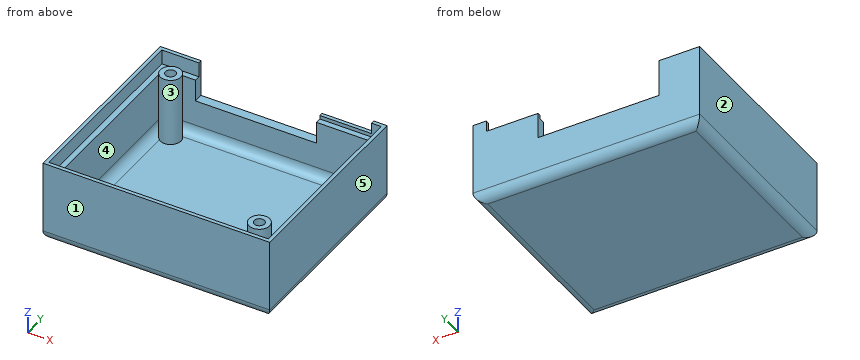
from build123d import *

# Parameters (mm, degrees)
F0_W        = 56.3
F0_H        = 48.55
F0_R        = 2.8
F1_DEPTH    = 2.5
F0_W_2      = 59.4
F0_H_2      = 51.65
F2_DEPTH    = 18
F0_W_3      = 61.4
F0_H_3      = 53.65
F3_DEPTH    = 22
F0_R_2      = 1.4
F4_DEPTH    = 21
F5_DEPTH    = 15
F6_T1_DEPTH = 48.55
F6_T3_DEPTH = 56.3
F6_T5_DEPTH = 73.9
F6_T7_DEPTH = 66.15
F7_W        = 32.75
F7_H        = 1
F7_H_2      = 1.55
F8_DEPTH    = 10
F7_W_2      = 14
F9_DEPTH    = 3


# Not quite as in the source:
# - a fillet or chamfer that OpenCascade refuses, or shapes differently, is made with other operations: its cross-section is extruded or revolved along the edge and cut away or added


with BuildPart() as f1:
    # F0 (on Top) → F1 (new body)
    with BuildSketch(Plane.XY):
        Rectangle(F0_W, F0_H)
        with Locations((23.88, -20.035)):
            Circle(F0_R, mode=Mode.SUBTRACT)
        with Locations((-23.91, 20.085)):
            Circle(F0_R, mode=Mode.SUBTRACT)
    extrude(amount=F1_DEPTH)

    # F0 (on Top) → F2 (join)
    with BuildSketch(Plane.XY):
        Rectangle(F0_W_2, F0_H_2)
        Rectangle(F0_W, F0_H, mode=Mode.SUBTRACT)
    extrude(amount=F2_DEPTH)

    # F0 (on Top) → F3 (join)
    with BuildSketch(Plane.XY):
        Rectangle(F0_W_3, F0_H_3)
        Rectangle(F0_W_2, F0_H_2, mode=Mode.SUBTRACT)
    extrude(amount=F3_DEPTH)

    # F0 (on Top) → F4 (join)
    with BuildSketch(Plane.XY):
        with Locations((-23.91, 20.085)):
            Circle(F0_R)
        with Locations((-23.91, 20.085)):
            Circle(F0_R_2, mode=Mode.SUBTRACT)
        with Locations((23.88, -20.035)):
            Circle(F0_R)
        with Locations((23.88, -20.035)):
            Circle(F0_R_2, mode=Mode.SUBTRACT)
    extrude(amount=F4_DEPTH)

    # F0 (on Top) → F5 (join)
    with BuildSketch(Plane.XY):
        with Locations((23.88, -20.035)):
            Circle(F0_R_2)
        with Locations((-23.91, 20.085)):
            Circle(F0_R_2)
    extrude(amount=F5_DEPTH)

    # F6: fillet of radius 2.5 on 8 edges, made by hand

    # F6_s2 → F6_t1 (join)
    with BuildSketch(Plane.XZ.offset(-24.275)):
        with BuildLine():
            ThreePointArc((28.15, 5), (27.417766953, 3.232233047), (25.65, 2.5))
            Line((25.65, 2.5), (28.15, 2.5))
            Line((28.15, 2.5), (28.15, 5))
        make_face()
        with BuildLine():
            ThreePointArc((-28.15, 5), (-27.417766953, 3.232233047), (-25.65, 2.5))
            Line((-25.65, 2.5), (-28.15, 2.5))
            Line((-28.15, 2.5), (-28.15, 5))
        make_face()
    extrude(amount=F6_T1_DEPTH)

    # F6_s4 → F6_t3 (join)
    with BuildSketch(Plane.YZ.offset(-28.15)):
        with BuildLine():
            ThreePointArc((24.275, 5), (23.542766953, 3.232233047), (21.775, 2.5))
            Line((21.775, 2.5), (24.275, 2.5))
            Line((24.275, 2.5), (24.275, 5))
        make_face()
        with BuildLine():
            ThreePointArc((-24.275, 5), (-23.542766953, 3.232233047), (-21.775, 2.5))
            Line((-21.775, 2.5), (-24.275, 2.5))
            Line((-24.275, 2.5), (-24.275, 5))
        make_face()
    extrude(amount=F6_T3_DEPTH)

    # F6_s6 → F6_t5 (cut)
    with BuildSketch(Plane.YZ.offset(-36.95)):
        with BuildLine():
            ThreePointArc((-24.325, 0), (-26.092766953, 0.732233047), (-26.825, 2.5))
            Line((-26.825, 2.5), (-26.825, 0))
            Line((-26.825, 0), (-24.325, 0))
        make_face()
        with BuildLine():
            ThreePointArc((24.325, 0), (26.092766953, 0.732233047), (26.825, 2.5))
            Line((26.825, 2.5), (26.825, 0))
            Line((26.825, 0), (24.325, 0))
        make_face()
    extrude(amount=F6_T5_DEPTH, mode=Mode.SUBTRACT)

    # F6_s8 → F6_t7 (cut)
    with BuildSketch(Plane.XZ.offset(-33.075)):
        with BuildLine():
            ThreePointArc((28.2, 0), (29.967766953, 0.732233047), (30.7, 2.5))
            Line((30.7, 2.5), (30.7, 0))
            Line((30.7, 0), (28.2, 0))
        make_face()
        with BuildLine():
            ThreePointArc((-28.2, 0), (-29.967766953, 0.732233047), (-30.7, 2.5))
            Line((-30.7, 2.5), (-30.7, 0))
            Line((-30.7, 0), (-28.2, 0))
        make_face()
    extrude(amount=F6_T7_DEPTH, mode=Mode.SUBTRACT)

    # F7 (on face) → F8 (cut)
    with BuildSketch(Plane.XY.offset(22)):
        with Locations((-3.275, 26.325)):
            Rectangle(F7_W, F7_H)
        with Locations((-3.275, 25.05)):
            Rectangle(F7_W, F7_H_2)
    extrude(amount=-F8_DEPTH, mode=Mode.SUBTRACT)

    # F7 (on face) → F9 (cut)
    with BuildSketch(Plane.XY.offset(22)):
        with Locations((20.1, 26.325)):
            Rectangle(F7_W_2, F7_H)
        with Locations((20.1, 25.05)):
            Rectangle(F7_W_2, F7_H_2)
    extrude(amount=-F9_DEPTH, mode=Mode.SUBTRACT)


solid = f1.part
The listing builds one solid part. Answer for the finished solid, in the listing's coordinates (mm). Face numbers are marked on the shaded views. A direction names the side the tool comes from. Round coordinates to 2 decimals unless told otherwise and drop trailing zeros. Order: outer loops, then holes, each group sorted by start corner. A loop starts at its lowest first (then second) coordinate and runs counter-clockwise, first axis right, second up. Notation, with made-up numbers: M 37.5,-34.5 L 61.5,-34.5 A18 ccw 61.5,-22.5 Z; hole C 32,-17 d11. An arc over 180 degrees is marked long. Answer in a Markdown table with one row per item. Add a question column.
1) Flat-ended cylindrical pins translate along their axes: pin 1 Ø1 at (x, z) = (-4.5, 13) entering from +Y (3 decimals); pin 2 Ø13 at (x, y) = (-5, 2) entering from +Z; pin 3 Ø0.5 at (x, y) = (19.5, 26.5) entering from +Z. Find the tip coordinate at first contact, or state that the pin passes through.
2) The part is cut by section C-C on x = 23.88. Determine the outline of the cut face in (y, z) (3 decimals), plus the area to 3 significant figures.
3) Consider line 1 along Y through (x, z) = (-23.91, 18.7) (3 decimals); line 2 along X through (y, z) = (20, 17.5); line 3 along Y through (x, z) = (-23.91, 17.05) (3 decimals). Determine where each line is inside the solid, lowest interval first. Write a range as from..to.
4) Which of the six approach directions +Z, -Z, +X, -X, +Y, -Y give full straight-line access (tool end or side, diameter ignored) to the marked faces 4 and 5?
5) Determine the mould class of the marked faces 1, 2 and 3 for opening direction Y: pulls with the +Y half, pulls with the -Y half, needs draft (parallel to the pull), parting line crosses it, or undercut.
6) The part is cut by section D-D on x = -23.91. Determine the outline of the cut face in (y, z) (3 decimals), plus the area to 3 significant figures.
7) The part is cut by section A-A on x = 8. Determine the outline of the cut face in (y, z) (3 decimals).
8) The part is cut by section B-B on y = 16.5. Determine the outline of the cut face in (x, z), plus the area to 3 significant figures.
Findings below:
| question | item | result |
|---|---|---|
| 1 | pin 1 | stops at y = -24.275 |
| 1 | pin 2 | stops at z = 2.5 |
| 1 | pin 3 | stops at z = 19 |
| 2 | outline | M -26.825,2.5 A2.5 ccw -24.325,0 L 24.325,0 A2.5 ccw 26.825,2.5 L 26.825,19 L 25.825,19 L 25.825,18 L 24.275,18 L 24.275,5 A2.5 cw 21.775,2.5 L -17.235,2.5 L -17.235,21 L -18.635,21 L -18.635,15 L -21.435,15 L -21.435,21 L -22.835,21 L -22.835,2.736 A2.5 cw -24.275,5 L -24.275,18 L -25.825,18 L -25.825,22 L -26.825,22 Z |
| 2 | area | 305 mm² |
| 3 | line 1 | y = -26.825..-25.825, 17.285..18.685, 21.485..22.885, 25.825..26.825 |
| 3 | line 2 | x = -30.7..-28.15, -26.71..-25.31, -22.51..-21.11, 28.15..30.7 |
| 3 | line 3 | y = -26.825..-24.275, 17.285..18.685, 21.485..22.885, 24.275..26.825 |
| 4 | face 4 | +Z |
| 4 | face 5 | +Z, -Z, +X, +Y, -Y |
| 5 | face 1 | pulls with the -Y half |
| 5 | face 2 | needs draft |
| 5 | face 3 | undercut |
| 6 | outline | M -26.825,2.5 A2.5 ccw -24.325,0 L 24.325,0 A2.5 ccw 26.825,2.5 L 26.825,22 L 25.825,22 L 25.825,18 L 24.275,18 L 24.275,5 A2.5 cw 22.885,2.76 L 22.885,21 L 21.485,21 L 21.485,15 L 18.685,15 L 18.685,21 L 17.285,21 L 17.285,2.5 L -21.775,2.5 A2.5 cw -24.275,5 L -24.275,18 L -25.825,18 L -25.825,22 L -26.825,22 Z |
| 6 | area | 308 mm² |
| 7 | outline | M -26.825,2.5 A2.5 ccw -24.325,0 L 24.325,0 A2.5 ccw 26.825,2.5 L 26.825,12 L 24.275,12 L 24.275,5 A2.5 cw 21.775,2.5 L -21.775,2.5 A2.5 cw -24.275,5 L -24.275,18 L -25.825,18 L -25.825,22 L -26.825,22 Z |
| 8 | outline | M -30.7,2.5 A2.5 ccw -28.2,0 L 28.2,0 A2.5 ccw 30.7,2.5 L 30.7,22 L 29.7,22 L 29.7,18 L 28.15,18 L 28.15,5 A2.5 cw 25.65,2.5 L -25.65,2.5 A2.5 cw -28.15,5 L -28.15,18 L -29.7,18 L -29.7,22 L -30.7,22 Z |
| 8 | area | 241 mm² |
